Read the model definition and answer for the solid it produces. Units are mm, in the model's axes. Face numbers are marked on the shaded views. A direction names the side the tool comes from. Give positions to 0.01 mm unless a question says otherwise; leave off trailing zeros. Write each loop counter-clockwise with the first axis right and the second up, starting at its lowest first coordinate (ties: lowest second). Pieces come first, ordered by that corner, then holes. Notation, with made-up numbers: M -30.75,87.25 L -3.75,87.25 A25 ccw -3.75,106.25 Z; hole C 43.5,-39.75 d4. An arc over 180 degrees is marked long. Put each result on its own line as item: value.
from build123d import *

# Parameters (mm, degrees)
SKETCH1_R           = 10
BOSS_EXTRUDE1_DEPTH = 50
SKETCH2_R           = 16.344073083
BOSS_EXTRUDE2_DEPTH = 10
CHAMFER1_SIZE       = 3
SKETCH3_OUTSIDE_W   = 48.308
SKETCH3_OUTSIDE_H   = 48.308
SKETCH3_OUTSIDE_R   = 9
CUT_EXTRUDE1_DEPTH  = 40


with BuildPart() as part:
    # Sketch1 → Boss-Extrude1 (new body)
    with BuildSketch(Plane.XY):
        Circle(SKETCH1_R)
    extrude(amount=BOSS_EXTRUDE1_DEPTH)

    # Sketch2 → Boss-Extrude2 (add)
    with BuildSketch(Plane(origin=(0, 0, 0), x_dir=(-1, 0, 0), z_dir=(0, 0, -1))):
        Circle(SKETCH2_R)
    extrude(amount=-BOSS_EXTRUDE2_DEPTH)

    # Chamfer1
    chamfer1_edges = [part.edges().sort_by_distance(p)[0] for p in [
        (-10, 0, 50),
    ]]
    chamfer(chamfer1_edges, length=CHAMFER1_SIZE)

    # Sketch3 outside → Cut-Extrude1 (cut)
    with BuildSketch(Plane.XY.offset(50)):
        Rectangle(SKETCH3_OUTSIDE_W, SKETCH3_OUTSIDE_H)
        Circle(SKETCH3_OUTSIDE_R, mode=Mode.SUBTRACT)
    extrude(amount=-CUT_EXTRUDE1_DEPTH, mode=Mode.SUBTRACT)


solid = part.part
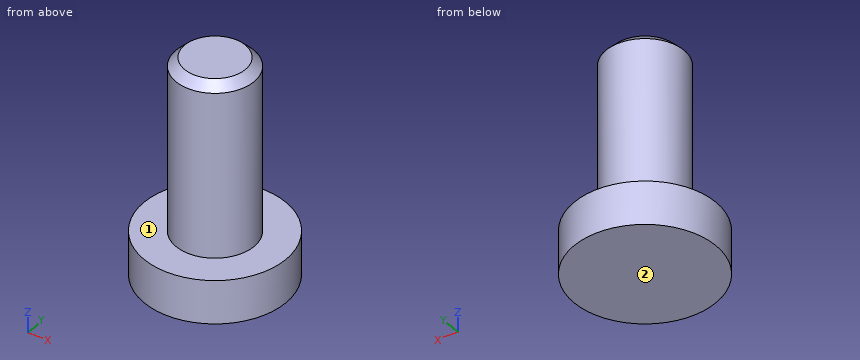
(1) Section C-C on z = 8 is taken. Determine the outline of the cut face in (x, y), and give its area (3 significant figures).
Result:
outline: C 0,0 d32.69
area: 839 mm²
(2) Section A-A on y = 0 is taken. Determine the outline of the cut face in (x, z), and give its area (3 significant figures).
Result:
outline: M -16.34,0 L 16.34,0 L 16.34,10 L 9,10 L 9,48 L 7,50 L -7,50 L -9,48 L -9,10 L -16.34,10 Z
area: 1,040 mm²
(3) Given pin 1 Ø12 at (y, z) = (-0.5, 28) entering from -X; pin 2 Ø12 at (y, z) = (7, 17.5) entering from -X; pin 3 Ø2 at (x, y) = (3, 8.5) entering from +Z, each flat-ended and moving along its own axis, determine where each tip first touches the part or whether it passes through.
Result:
pin 1: stops at x = -9
pin 2: stops at x = -8.94
pin 3: stops at z = 48.99
(4) Straight lines are drawn through the part: line 1 along Z through (x, y) = (-4.5, -11); line 2 along Y through (x, z) = (-0.5, 8); line 3 along Y through (x, z) = (-11, 5.5). For each, find the intervals that lie inside material, in ascending order. Write a range as from..to.
Result:
line 1: z = 0..10
line 2: y = -16.34..16.34
line 3: y = -12.09..12.09
(5) Which of the six approach directions +Z, -Z, +X, -X, +Y, -Y give full straight-line access (tool end or side, diameter ignored) to the marked faces 1 and 2?
Result:
face 1: +Z
face 2: -Z, +X, -X, +Y, -Y
(6) Section D-D on x = 14 is taken. Determine the outline of the cut face in (y, z), and give its area (3 significant figures).
Result:
outline: M -8.43,0 L 8.43,0 L 8.43,10 L -8.43,10 Z
area: 169 mm²
